Job drawing, mm, ordinate dimensions from the low corner. One solid piece. Round coordinates to 2 decimals unless told otherwise and drop trailing zeros. Loops run counter-clockwise (first coordinate to the right, second up) from the corner with the lowest first, then second, coordinate; pieces in that order, holes last.
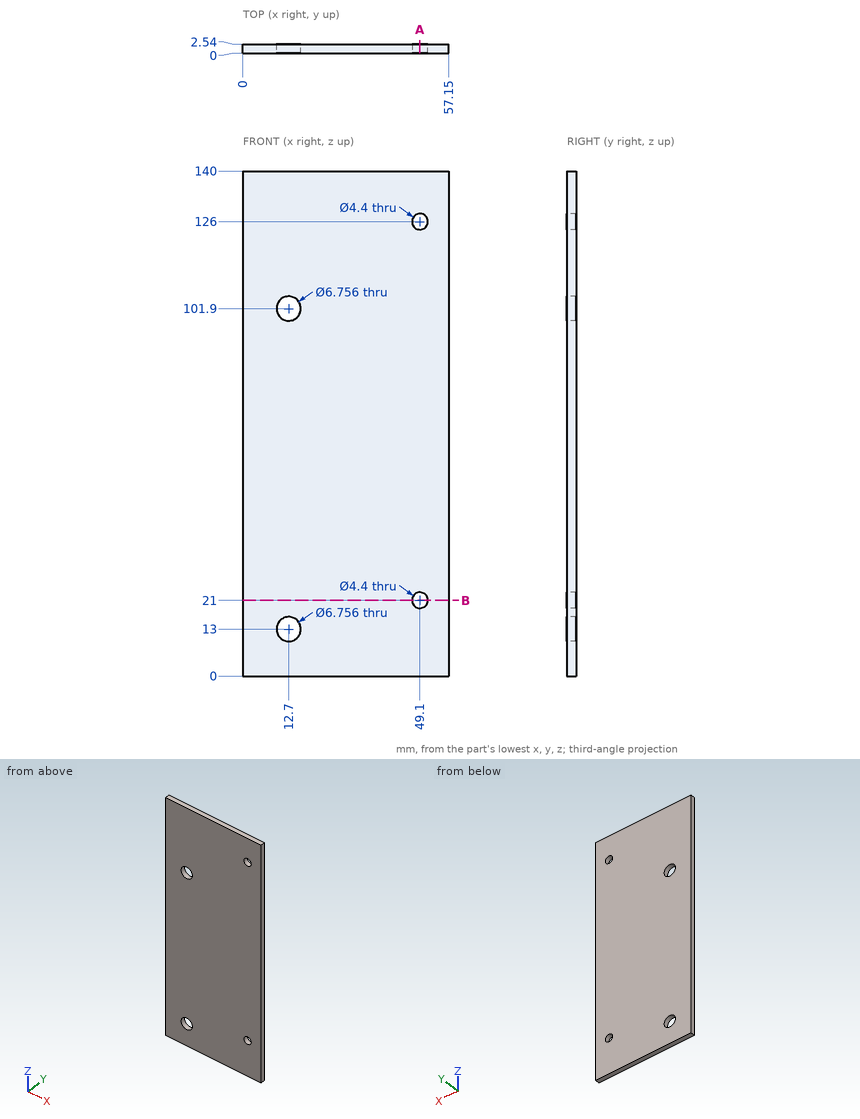
(1) Pin check, flat tip, straight feed: P1, Ø6, axis at x = 12.7, z = 101.9, coming from the -Y side. Stop position of the tip, or through.
Responses:
P1: passes through
(2) Slice it at A-A on x = 49.1. List the corners of the cut face in (y, z).
Responses:
outline: (0, 0) - (2.54, 0) - (2.54, 18.8) - (0, 18.8) - close; (0, 23.2) - (2.54, 23.2) - (2.54, 123.8) - (0, 123.8) - close; (0, 128.2) - (2.54, 128.2) - (2.54, 140) - (0, 140) - close
(3) Probe line 1 (Z direction, x = 49.1, y = 1.4); line 2 (X direction, y = 1.9, z = 126); line 3 (X direction, y = 2, z = 13). List the from-to ranges inside material, lowest first.
Responses:
line 1: z = 0 to 18.8, 23.2 to 123.8, 128.2 to 140
line 2: x = 0 to 46.9, 51.3 to 57.15
line 3: x = 0 to 9.32, 16.08 to 57.15
(4) Slice it at B-B on z = 21. List the corners of the cut face in (x, y), plus the area to 3 significant figures.
Responses:
outline: (0, 0) - (46.9, 0) - (46.9, 2.54) - (0, 2.54) - close; (51.3, 0) - (57.15, 0) - (57.15, 2.54) - (51.3, 2.54) - close
area: 134 mm2
